```python
from build123d import *

# Parameters (mm, degrees)
FILLET1_R = 3.175
FILLET2_R = 3.175
FILLET3_R = 3.175
FILLET4_R = 3.175


with BuildPart() as part:
    # Sketch1 → Revolve1 (revolve)
    with BuildSketch(Plane(origin=(0, 0, 0), x_dir=(0, 0, -1), z_dir=(1, 0, 0))):
        Polygon((-25.4, 12.7), (25.4, 12.7), (25.4, 17.78), (5.08, 17.78), (5.08, 39.878), (19.05, 44.958), (19.05, 50.038), (-19.05, 50.038), (-19.05, 44.958), (-5.08, 39.878), (-5.08, 17.78), (-25.4, 17.78), align=None)
    revolve(axis=Axis((0, 0, 55.673126484), (0, 0, -1)))

    # Fillet1
    fillet1_edges = [part.edges().sort_by_distance(p)[0] for p in [
        (0, -17.78, 5.08),
    ]]
    fillet(fillet1_edges, radius=FILLET1_R)

    # Fillet2
    fillet2_edges = [part.edges().sort_by_distance(p)[0] for p in [
        (0, -39.878, 5.08),
    ]]
    fillet(fillet2_edges, radius=FILLET2_R)

    # Fillet3
    fillet3_edges = [part.edges().sort_by_distance(p)[0] for p in [
        (0, -17.78, -5.08),
    ]]
    fillet(fillet3_edges, radius=FILLET3_R)

    # Fillet4
    fillet4_edges = [part.edges().sort_by_distance(p)[0] for p in [
        (0, -39.878, -5.08),
    ]]
    fillet(fillet4_edges, radius=FILLET4_R)


solid = part.part
```
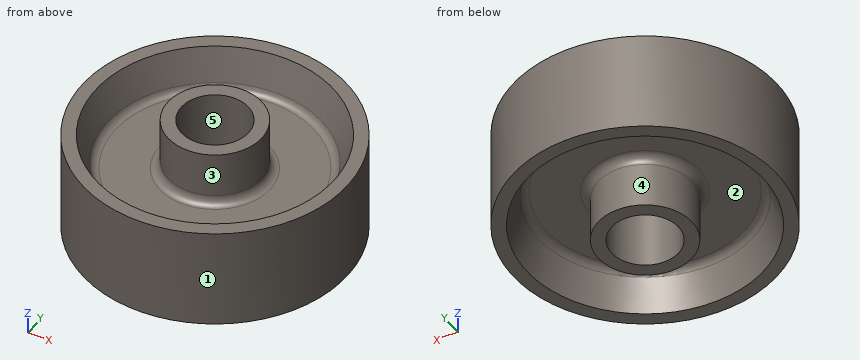
Design review of the part built by this model. Coordinates are the model's own, in mm. Face numbers are marked on the shaded views. A direction names the side the tool comes from. Coordinates: 2 decimals unless noted, no trailing zeros. Order: outer loops, then holes, each group sorted by start corner. A loop starts at its lowest first (then second) coordinate and runs counter-clockwise, first axis right, second up.
1) Clearance check with flat-ended pins moving along their axes: pin 1 (3 mm diameter, centred on y = -10, z = 9.5, fed in from -X); pin 2 (5 mm diameter, centred on x = -5, y = -24, fed in from +Z); pin 3 (10 mm diameter, centred on x = 8, z = 0, fed in from +Y). State where each tip first meets the part, or that it passes through.
2) Wall thickness on line 1 along Y through (x, z) = (-15, 8); line 2 along X through (y, z) = (3, -7); line 3 along X through (y, z) = (-7.5, 9.5): over which ranges is each line inside the solid? List them lowest first.
3) Mouldability with a two-part tool opening along Y and no side actions: class the marked faces 1 and 2 as +Y half, -Y half, draft (parallel to the pull), parting line (faces both ways), or undercut.
4) For the marked faces 3, 4 and 5, list the 3-axis set-ups (+Z, -Z, +X, -X, +Y, -Y) from which the entire face can be reached by the end or side of a thin tool; tool diameter is ignored.
5) Take a section at D-D, the plane z = 3. Give the boundary of the cut face in (x, y), and give its area (3 significant figures).
6) Take a section at C-C, the plane z = 13.5. Give the boundary of the cut face in (x, y).
Returned:
1. pin 1: stops at x = -49.31
1. pin 2: stops at z = 5.08
1. pin 3: stops at y = 49.95
2. line 1: y = -47.74 to -38.09, -9.57 to 9.57, 38.09 to 47.74
2. line 2: x = -49.95 to -40.46, -17.79 to -12.34, 12.34 to 17.79, 40.46 to 49.95
2. line 3: x = -49.47 to -40.8, -16.12 to -10.25, 10.25 to 16.12, 40.8 to 49.47
3. face 1: parting line
3. face 2: undercut
4. face 3: +Z
4. face 4: -Z
4. face 5: +Z, -Z
5. outline: circle Ø100.08 at (0, 0); hole circle Ø25.4 at (0, 0)
5. area: 7,360 mm2
6. outline: circle Ø100.08 at (0, 0); circle Ø35.56 at (0, 0); hole circle Ø85.88 at (0, 0); hole circle Ø25.4 at (0, 0)
